Design review of the part built by this model. Coordinates are the model's own, in mm. Face numbers are marked on the shaded views. Coordinates: 2 decimals unless noted, no trailing zeros. Order: outer loops, then holes, each group sorted by start corner. A loop starts at its lowest first (then second) coordinate and runs counter-clockwise, first axis right, second up. Notation, with made-up numbers: M 77,27.25 L 123,27.25 A13 ccw 123,40.25 Z; hole C -11.5,-31 d9. An arc over 180 degrees is marked long. Answer in a Markdown table with one row per item.
from build123d import *

# Parameters (mm, degrees)
SZKIC2_W                        = 14
SZKIC2_H                        = 14
DODANIE_WYCI_GNI_CIE1_DEPTH     = 4.5
WYTNIJ_WYCI_GNI_CIE1_DEPTH      = 11.062305899
WYTNIJ_WYCI_GNI_CIE1_DEPTH_BACK = 11.062305899
SZKIC7_R                        = 3
SFAZOWANIE1_SIZE                = 0.5


with BuildPart() as part:
    # Szkic2 → Dodanie-wyciągnięcie1 (new, symmetric)
    with BuildSketch(Plane.XY):
        Rectangle(SZKIC2_W, SZKIC2_H)
    extrude(amount=DODANIE_WYCI_GNI_CIE1_DEPTH, both=True)

    # Szkic6 → Wycięcie-obrót1 (revolve, cut)
    with BuildSketch(Plane(origin=(0, 0, 0), x_dir=(0, 0, -1), z_dir=(1, 0, 0))):
        with BuildLine():
            Line((0, 6.363961031), (0, 11.1169554))
            Line((0, 11.1169554), (-10.01359094, 11.1169554))
            Line((-10.01359094, 11.1169554), (-10.01359094, -12.11227334))
            Line((-10.01359094, -12.11227334), (0, -12.11227334))
            Line((0, -12.11227334), (0, -6.363961031))
            ThreePointArc((0, -6.363961031), (-6.363961031, 0), (0, 6.363961031))
        make_face()
    revolve(axis=Axis((0, -12.574301311, 0), (0, 1, 0)), mode=Mode.SUBTRACT)

    # Szkic7 → Wytnij-wyciągnięcie1 (cut, two sides: drawn at the far end of the back side and taken through both)
    with BuildSketch(Plane.XY.offset(-WYTNIJ_WYCI_GNI_CIE1_DEPTH_BACK)):
        Circle(SZKIC7_R)
    extrude(amount=WYTNIJ_WYCI_GNI_CIE1_DEPTH + WYTNIJ_WYCI_GNI_CIE1_DEPTH_BACK, mode=Mode.SUBTRACT)

    # Sfazowanie1
    sfazowanie1_edges = [part.edges().sort_by_distance(p)[0] for p in [
        (-3, 0, -4.5),
        (-3, 0, 4.5),
    ]]
    chamfer(sfazowanie1_edges, length=SFAZOWANIE1_SIZE)


solid = part.part
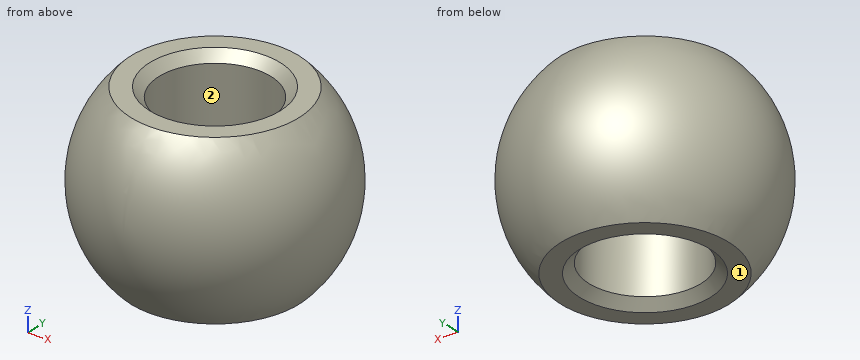
(1) Add section D-D, the plane z = 0.25. Give the boundary of the cut face in (x, y), and give its area (3 significant figures).
Return value:
| item | result |
|---|---|
| outline | C 0,0 d12.72; hole C 0,0 d6 |
| area | 98.8 mm2 |
(2) Draft analysis for pull direction X (two halves, no side actions). For the marked faces 1 and 2, state which applies: pulls with the +X half, pulls with the -X half, needs draft (parallel to the pull), parting line crosses it, or undercut.
Return value:
| item | result |
|---|---|
| face 1 | needs draft |
| face 2 | undercut |
(3) Add section A-A, the plane y = 0. Give the boundary of the cut face in (x, z).
Return value:
| item | result |
|---|---|
| outline | M -4.5,-4.5 L -3.5,-4.5 L -3,-4 L -3,4 L -3.5,4.5 L -4.5,4.5 A6.36 ccw Z; M 3,-4 L 3.5,-4.5 L 4.5,-4.5 A6.36 ccw 4.5,4.5 L 3.5,4.5 L 3,4 Z |
(4) Add section C-C, the plane z = 3.25. Give the boundary of the cut face in (x, y).
Return value:
| item | result |
|---|---|
| outline | C 0,0 d10.94; hole C 0,0 d6 |
(5) Insertion check: pin 1 Ø2 at (x, z) = (-4, -2) entering from -Y; pin 2 Ø1 at (y, z) = (-4, 3) entering from -X; pin 3 Ø2 at (x, z) = (1, 1.5) entering from +Y. Each pin has a flat end and moves straight along its axis. Give the tip position at first contact, or say it passes through.
Return value:
| item | result |
|---|---|
| pin 1 | stops at y = -5.33 |
| pin 2 | stops at x = -4.5 |
| pin 3 | stops at y = 6.31 |
(6) For line 1 along X through (y, z) = (0.5, -1); line 2 along Y through (x, z) = (0, -0.25); line 3 along Y through (x, z) = (0, -0.75), list the stretches that pass through material, from the lowest coordinate up. Write a range as from..to.
Return value:
| item | result |
|---|---|
| line 1 | x = -6.26..-2.96, 2.96..6.26 |
| line 2 | y = -6.36..-3, 3..6.36 |
| line 3 | y = -6.32..-3, 3..6.32 |
